Part model, mm, in its own coordinate system. Face numbers are marked on the shaded views. A direction names the side the tool comes from. Give positions to 0.01 mm unless a question says otherwise; leave off trailing zeros. Order: outer loops, then holes, each group sorted by start corner. A loop starts at its lowest first (then second) coordinate and runs counter-clockwise, first axis right, second up. Notation, with made-up numbers: M -12,71.25 L -2,71.25 A14 cw -2,81.25 Z; hole C 20.5,3 d11. An arc over 180 degrees is marked long. Return JSON: item names as keys, results as strings.
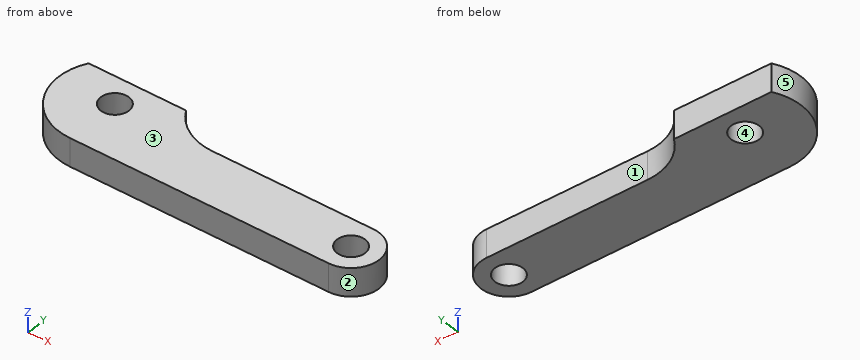
from build123d import *

# Parameters (mm, degrees)
ESQUISSE1_R             = 2.5
BOSS_EXTRU_1_DEPTH      = 5
CONG_1_R                = 10
ESQUISSE2_W             = 18.660254038
ESQUISSE2_H             = 5
ENL_V_MAT_EXTRU_1_DEPTH = 5


with BuildPart() as part:
    # Esquisse1 → Boss.-Extru.1 (new body)
    with BuildSketch(Plane.XY):
        with BuildLine():
            Line((0, 0), (-46, 0))
            ThreePointArc((-46, 0), (-53.071067812, 17.071067812), (-36, 10))
            Line((-36, 10), (0, 10))
            ThreePointArc((0, 10), (5, 5), (0, 0))
        make_face()
        with Locations((-46, 10)):
            Circle(ESQUISSE1_R, mode=Mode.SUBTRACT)
        with Locations((0, 5)):
            Circle(ESQUISSE1_R, mode=Mode.SUBTRACT)
    extrude(amount=BOSS_EXTRU_1_DEPTH)

    # Congé1
    cong_1_edges = [part.edges().sort_by_distance(p)[0] for p in [
        (-36, 10, 2.5),
    ]]
    fillet(cong_1_edges, radius=CONG_1_R)

    # Esquisse2 → Enlèv. mat.-Extru.1 (cut)
    with BuildSketch(Plane.XY.offset(5)):
        with Locations((-46.669872981, 17.5)):
            Rectangle(ESQUISSE2_W, ESQUISSE2_H)
    extrude(amount=-ENL_V_MAT_EXTRU_1_DEPTH, mode=Mode.SUBTRACT)


solid = part.part
Q1. Band-saw the part on C-C (x = -3.5). Give the cut face in (y, z).
Established:
{"outline": "M 0,0 L 10,0 L 10,5 L 0,5 Z"}
Q2. Pin check, flat tips, straight feed: pin 1 (2 mm diameter, centred on x = -32, z = 3.5, fed in from -Y); pin 2 (2 mm diameter, centred on y = 5.5, z = 0.5, fed in from -X). Stop position of each tip, or through.
Established:
{"pin 1": "stops at y = 0", "pin 2": "stops at x = -55.37"}
Q3. Band-saw the part on A-A (y = 5). Give the cut face in (x, z), then the cut area to 3 significant figures.
Established:
{"outline": "M -54.66,0 L -2.5,0 L -2.5,5 L -54.66,5 Z; M 2.5,0 L 5,0 L 5,5 L 2.5,5 Z", "area": "273 mm²"}
Q4. Two-plate mould, pull along Y, no slides. Class the marked faces 3, 4 and 5: +Y half, -Y half, draft (parallel to the pull), parting line (faces both ways), or undercut.
Established:
{"face 3": "draft", "face 4": "undercut", "face 5": "parting line"}
Q5. Band-saw the part on B-B (z = 2.1). Give the cut face in (x, y), then the cut area to 3 significant figures.
Established:
{"outline": "M -54.66,15 A10 ccw -46,0 L 0,0 A5 ccw 0,10 L -28.68,10 A10 cw -37.34,15 Z; hole C -46,10 d5; hole C 0,5 d5", "area": "642 mm²"}
Q6. Probe line 1 along Y through (x, z) = (-46, 3.5); line 2 along Y through (x, z) = (-14.5, 4.7); line 3 along X through (y, z) = (5.5, 3.95). List the from-to ranges inside material, lowest first.
Established:
{"line 1": "y = 0 to 7.5, 12.5 to 15", "line 2": "y = 0 to 10", "line 3": "x = -54.93 to -2.45, 2.45 to 4.97"}
Q7. Band-saw the part on D-D (y = 13.75). Give the cut face in (x, z), then the cut area to 3 significant figures.
Established:
{"outline": "M -55.27,0 L -36.49,0 L -36.49,5 L -55.27,5 Z", "area": "93.9 mm²"}
Q8. 3-axis set-ups, long thin cutter, end or side, ignore diameter. For the marked faces 1 and 2: which of +Z, -Z, +X, -X, +Y, -Y reach the whole face in a straight line?
Established:
{"face 1": "+Z, -Z, +X, +Y", "face 2": "+Z, -Z, +X"}
